from build123d import *

# Parameters (mm, degrees)
SKETCH1_W                 = 35
SKETCH1_H                 = 27.36
SKETCH1_R                 = 4
BOSS_EXTRUDE1_DEPTH       = 5.5
BOSS_EXTRUDE2_START       = -11.5
BOSS_EXTRUDE2_OUTLINE_W   = 35
BOSS_EXTRUDE2_OUTLINE_H   = 47.36
BOSS_EXTRUDE2_OUTLINE_R   = 4
BOSS_EXTRUDE2_OUTLINE_R_2 = 2.3
BOSS_EXTRUDE2_DEPTH       = 6
FILLET1_R                 = 5
CUT_EXTRUDE1_DEPTH        = 15
CUT_EXTRUDE1_DEPTH_BACK   = 42.689562243
SKETCH4_R                 = 1.4
CUT_EXTRUDE2_START        = -6
SKETCH4_3_R               = 3.5
SKETCH4_3_R_2             = 1.4
CUT_EXTRUDE2_DEPTH        = 15


# Read off the part's stored shape, not the designer's step: Boss-Extrude2
with BuildPart() as part:
    # Sketch1 → Boss-Extrude1 (new body)
    with BuildSketch(Plane(origin=(0, 0, 0), x_dir=(1, 0, 0), z_dir=(0, 1, 0))):
        with Locations((0, 12.715830395)):
            Rectangle(SKETCH1_W, SKETCH1_H)
        with Locations(Location((0, 9.035830395, 0), (0, 0, 270))):
            Circle(SKETCH1_R, mode=Mode.SUBTRACT)
    extrude(amount=BOSS_EXTRUDE1_DEPTH)

    # Boss-Extrude2 outline → Boss-Extrude2 (add)
    with BuildSketch(Plane(origin=(0, 5.5, 0), x_dir=(1, 0, 0), z_dir=(0, 1, 0)).offset(BOSS_EXTRUDE2_START)):
        with Locations((0, 22.715830395)):
            Rectangle(BOSS_EXTRUDE2_OUTLINE_W, BOSS_EXTRUDE2_OUTLINE_H)
        with Locations((0, 9.035830395)):
            Circle(BOSS_EXTRUDE2_OUTLINE_R, mode=Mode.SUBTRACT)
        with Locations((-9.5, 36.395830395)):
            Circle(BOSS_EXTRUDE2_OUTLINE_R_2, mode=Mode.SUBTRACT)
        with Locations((9.5, 36.395830395)):
            Circle(BOSS_EXTRUDE2_OUTLINE_R_2, mode=Mode.SUBTRACT)
    extrude(amount=BOSS_EXTRUDE2_DEPTH)

    # Fillet1
    fillet1_edges = [part.edges().sort_by_distance(p)[0] for p in [
        (17.5, -3, 0.964169605),
        (-17.5, -3, 0.964169605),
    ]]
    fillet(fillet1_edges, radius=FILLET1_R)

    # Sketch4 → Cut-Extrude1 (cut, two sides: drawn at the far end of the back side and taken through both)
    with BuildSketch(Plane(origin=(0, 0, -9.035830395), x_dir=(-1, 0, 0), z_dir=(0, 0, -1)).offset(-CUT_EXTRUDE1_DEPTH_BACK)):
        with Locations((-11.980167066, 0.5)):
            Circle(SKETCH4_R)
        with Locations((11.980167066, 0.5)):
            Circle(SKETCH4_R)
    extrude(amount=CUT_EXTRUDE1_DEPTH + CUT_EXTRUDE1_DEPTH_BACK, mode=Mode.SUBTRACT)

    # Sketch4<3> → Cut-Extrude2 (cut)
    # profile 1 of 2: a face of its own
    with BuildSketch(Plane(origin=(0, 0, -9.035830395), x_dir=(-1, 0, 0), z_dir=(0, 0, -1)).offset(CUT_EXTRUDE2_START)):
        with Locations((-11.980167066, 0.5)):
            Circle(SKETCH4_3_R)
        with Locations((-11.980167066, 0.5)):
            Circle(SKETCH4_3_R_2, mode=Mode.SUBTRACT)
    # profile 2 of 2: a face of its own
    with BuildSketch(Plane(origin=(0, 0, -9.035830395), x_dir=(-1, 0, 0), z_dir=(0, 0, -1)).offset(CUT_EXTRUDE2_START)):
        with Locations((11.980167066, 0.5)):
            Circle(SKETCH4_3_R)
        with Locations((11.980167066, 0.5)):
            Circle(SKETCH4_3_R_2, mode=Mode.SUBTRACT)
    extrude(amount=-CUT_EXTRUDE2_DEPTH, mode=Mode.SUBTRACT)


solid = part.part
Work out the finished part from the listing and answer in its coordinate system (mm). A direction names the side the tool comes from. Give positions to 0.01 mm unless a question says otherwise; leave off trailing zeros. Write each loop counter-clockwise with the first axis right and the second up, starting at its lowest first coordinate (ties: lowest second). Pieces come first, ordered by that corner, then holes.
Q1. The part is cut by section B-B on y = 1. Give the vertices of the cut face in (x, z).
Answer:
outline: (-17.5, -26.4) - (17.5, -26.4) - (17.5, -4.04) arc R5 ccw to (15.44, 0.01) - (15.44, -3.04) - (13.29, -3.04) - (13.29, -24.04) - (10.67, -24.04) - (10.67, -3.04) - (8.52, -3.04) - (8.52, 0.96) - (-8.52, 0.96) - (-8.52, -3.04) - (-10.67, -3.04) - (-10.67, -24.04) - (-13.29, -24.04) - (-13.29, -3.04) - (-15.44, -3.04) - (-15.44, 0.01) arc R5 ccw to (-17.5, -4.04) - close; hole circle Ø8 at (0, -9.04)
Q2. Straight lines are drawn through the part: L1, parallel to Y at x = -12, z = -16; L2, parallel to Z at x = 0, y = 0.5; L3, parallel to X at y = 2.5, z = -3. For each, find the intervals that lie inside material, in ascending order.
Answer:
L1: y = -6 to -0.9, 1.9 to 5.5
L2: z = -26.4 to -13.04, -5.04 to 0.96
L3: x = -17.39 to -14.85, -9.11 to 9.11, 14.85 to 17.39
Q3. The part is cut by section A-A on z = -15. Give the vertices of the cut face in (x, y), and give its area (3 significant figures).
Answer:
outline: (-17.5, -6) - (17.5, -6) - (17.5, 5.5) - (-17.5, 5.5) - close; hole circle Ø2.8 at (-11.98, 0.5); hole circle Ø2.8 at (11.98, 0.5)
area: 390 mm2
Q4. The part is cut by section C-C on x = -2. Give the vertices of the cut face in (y, z).
Answer:
outline: (-6, -46.4) - (0, -46.4) - (0, -26.4) - (5.5, -26.4) - (5.5, -12.5) - (-6, -12.5) - close; (-6, -5.57) - (5.5, -5.57) - (5.5, 0.96) - (-6, 0.96) - close
Q5. A tool of negligible diameter and unlimited length cuts with its end or side. For faces 4 (the face through (-8.484, 0.654, -1.064)), 5 (the face through (3.5, 0.9, -7.1)), 6 (the face through (0, 0, -37)), from which of +Z, -Z, +X, -X, +Y, -Y can it reach the whole face along a straight path? Write none if from no direction.
Answer:
face 4: +Z
face 5: +Y, -Y
face 6: -Z, +X, -X, +Y
Q6. Given pin 1 (3 mm diameter, centred on x = -0.5, z = -33.5, fed in from +Y); pin 2 (1.7 mm diameter, centred on x = -11.98, y = 0.5, fed in from +Z); pin 3 (2 mm diameter, centred on x = 12, y = 0, fed in from +Z); pin 4 (3.5 mm diameter, centred on x = 9.5, z = -36.4, fed in from -Y), each flat-ended and moving along its own axis, determine where each tip first touches the part or whether it passes through.
Answer:
pin 1: stops at y = 0
pin 2: stops at z = -24.04
pin 3: stops at z = -3.04
pin 4: passes through
Q7. For a pull along Y with two mould halves and no side action, classify faces 1 (the face through (0, -3, -46.396)), 2 (the face through (0, 5.5, -16)), 3 (the face through (-13.316, 0.921, -13.389)) as released by +Y, released by -Y, zero draft, split by the parting line, or undercut.
Answer:
face 1: zero draft
face 2: released by +Y
face 3: undercut
Q8. The part is cut by section D-D on y = -4.5. Give the vertices of the cut face in (x, z), and give its area (3 significant figures).
Answer:
outline: (-17.5, -46.4) - (17.5, -46.4) - (17.5, -4.04) arc R5 ccw to (12.5, 0.96) - (-12.5, 0.96) arc R5 ccw to (-17.5, -4.04) - close; hole circle Ø4.6 at (-9.5, -36.4); hole circle Ø8 at (0, -9.04); hole circle Ø4.6 at (9.5, -36.4)
area: 1,560 mm2
